The listing builds one solid part. Answer for the finished solid, in the listing's coordinates (mm). A direction names the side the tool comes from. Coordinates: 2 decimals unless noted, no trailing zeros. Loops run counter-clockwise (first coordinate to the right, second up) from the corner with the lowest first, then second, coordinate; pieces in that order, holes last. Notation, with made-up numbers: M 34,81 L 90,81 A10 cw 90,92 Z; hole C -1,-35 d11. An arc over 180 degrees is marked long. Answer as a JSON object with one key per item and string values. Group by question number.
1. A cutting plane is placed at B-B on x = 0. State how many separate pieces and enclosed holes the cut face has, and give its area (3 significant figures).
2. A cutting plane is placed at A-A on z = -19.05. Give the vertices of the cut face in (x, y) (3 decimals).
3. Straight lines are drawn through the part: L1, parallel to X at y = -11, z = 19; L2, parallel to X at y = 54, z = 12.5; L3, parallel to X at y = -44, z = 22. For each, find the intervals that lie inside material, in ascending order.
4. A cutting plane is placed at C-C on y = 31. Give the vertices of the cut face in (x, z).
5. Determine the mould class of faces 4 (the face through (0, -44, 19.3)), 5 (the face through (0, 1, 25.4)), 6 (the face through (0.044, -22.263, -18.706)) for opening direction Z: released by +Z, released by -Z, zero draft, split by the parting line, or undercut.
6. Given pin 1 (3 mm diameter, centred on x = 7.79, y = -31.24, fed in from +Z); pin 2 (2 mm diameter, centred on x = 14, z = 20.5, fed in from +Y); pin 3 (12 mm diameter, centred on x = -6, z = -10, fed in from +Y); pin 4 (8 mm diameter, centred on x = 13.5, z = 20.5, fed in from +Y), each flat-ended and moving along its own axis, determine where each tip first touches the part or whether it passes through.
7. For faces 1 (the face through (0, 56.059, 13)), 2 (the face through (12.7, 10, 12)), 3 (the face through (-8.11, -24.44, -12.52)), determine the directions among +Z, -Z, +X, -X, +Y, -Y from which every point of the face is accessible in a straight line to the end or side of a thin tool.
8. A cutting plane is placed at D-D on y = -39.5. Give the vertices of the cut face in (x, z), and give its area (3 significant figures).
from build123d import *

# Parameters (mm, degrees)
SKETCH1_R           = 4
SKETCH1_R_2         = 0.762
BOSS_EXTRUDE1_DEPTH = 25.4
SKETCH2_R           = 19.05
BOSS_EXTRUDE2_DEPTH = 25.4
SKETCH5_R           = 6.35
CUT_EXTRUDE2_DEPTH  = 25.4
SKETCH3_R           = 1.6
CUT_EXTRUDE1_DEPTH  = 25.4
SKETCH6_W           = 3.175
SKETCH6_H           = 1.5875
CUT_EXTRUDE3_DEPTH  = 25.4
SKETCH8_R           = 19.05
CUT_EXTRUDE4_DEPTH  = 19.3
BOSS_EXTRUDE3_DEPTH = 25.4
SKETCH10_W          = 6.35
SKETCH10_H          = 4.7625
BOSS_EXTRUDE4_DEPTH = 25.4
SKETCH11_R          = 1.5875
CUT_EXTRUDE5_DEPTH  = 23.225


with BuildPart() as part:
    # Sketch1 → Boss-Extrude1 (new body)
    with BuildSketch(Plane.XY):
        with BuildLine():
            Line((12.7, 50.8), (12.7, -50.8))
            ThreePointArc((12.7, -50.8), (0, -63.5), (-12.7, -50.8))
            Line((-12.7, -50.8), (-12.7, 50.8))
            ThreePointArc((-12.7, 50.8), (0, 63.5), (12.7, 50.8))
        make_face()
        with Locations((0, 50.8)):
            Circle(SKETCH1_R, mode=Mode.SUBTRACT)
        with Locations((-5.118745989, 55.918745989)):
            Circle(SKETCH1_R_2, mode=Mode.SUBTRACT)
        with Locations((5.118745989, 55.918745989)):
            Circle(SKETCH1_R_2, mode=Mode.SUBTRACT)
        with Locations((5.118745989, 45.681254011)):
            Circle(SKETCH1_R_2, mode=Mode.SUBTRACT)
        with Locations((-5.118745989, 45.681254011)):
            Circle(SKETCH1_R_2, mode=Mode.SUBTRACT)
    extrude(amount=BOSS_EXTRUDE1_DEPTH)

    # Sketch2 → Boss-Extrude2 (add)
    with BuildSketch(Plane(origin=(0, 0, 0), x_dir=(-1, 0, 0), z_dir=(0, 0, -1))):
        with Locations((0, -44.45)):
            Circle(SKETCH2_R)
    extrude(amount=-BOSS_EXTRUDE2_DEPTH)

    # Sketch5 → Cut-Extrude2 (cut)
    with BuildSketch(Plane.XY.offset(25.4)):
        with Locations((0, -51.562)):
            Circle(SKETCH5_R)
    extrude(amount=-CUT_EXTRUDE2_DEPTH, mode=Mode.SUBTRACT)

    # Sketch3 → Cut-Extrude1 (cut)
    with BuildSketch(Plane.XY.offset(25.4)):
        with Locations((-7.794229315, -31.235903463)):
            Circle(SKETCH3_R)
        with Locations((-15.2766, -44.45)):
            Circle(SKETCH3_R)
        with Locations((15.2766, -44.45)):
            Circle(SKETCH3_R)
        with Locations((-7.794229315, -58.017540858)):
            Circle(SKETCH3_R)
        with Locations((7.794229315, -31.235903463)):
            Circle(SKETCH3_R)
        with Locations((7.794229315, -58.017540858)):
            Circle(SKETCH3_R)
    extrude(amount=-CUT_EXTRUDE1_DEPTH, mode=Mode.SUBTRACT)

    # Sketch6 → Cut-Extrude3 (cut)
    with BuildSketch(Plane(origin=(0, 0, 0), x_dir=(-1, 0, 0), z_dir=(0, 0, -1))):
        with Locations((0, 55.265240671)):
            Rectangle(SKETCH6_W, SKETCH6_H)
    extrude(amount=-CUT_EXTRUDE3_DEPTH, mode=Mode.SUBTRACT)

    # Sketch8 → Cut-Extrude4 (cut)
    with BuildSketch(Plane(origin=(0, 0, 0), x_dir=(-1, 0, 0), z_dir=(0, 0, -1))):
        with Locations((0, -44.45)):
            Circle(SKETCH8_R)
    extrude(amount=-CUT_EXTRUDE4_DEPTH, mode=Mode.SUBTRACT)

    # Sketch9 → Boss-Extrude3 (add)
    with BuildSketch(Plane(origin=(0, 0, 0), x_dir=(-1, 0, 0), z_dir=(0, 0, -1))):
        with BuildLine():
            Line((-12.7, -30.250968343), (-12.7, -26.990386602))
            ThreePointArc((-12.7, -26.990386602), (0, -22.86), (12.7, -26.990386602))
            Line((12.7, -26.990386602), (12.7, -30.250968343))
            ThreePointArc((12.7, -30.250968343), (0, -25.4), (-12.7, -30.250968343))
        make_face()
    extrude(amount=BOSS_EXTRUDE3_DEPTH)

    # Sketch10 → Boss-Extrude4 (add)
    with BuildSketch(Plane(origin=(0, 0, 0), x_dir=(-1, 0, 0), z_dir=(0, 0, -1))):
        with Locations((0, -20.713481915)):
            Rectangle(SKETCH10_W, SKETCH10_H)
    extrude(amount=BOSS_EXTRUDE4_DEPTH)

    # Sketch11 → Cut-Extrude5 (cut, through all)
    with BuildSketch(Plane(origin=(3.175, 0, 0), x_dir=(0, 0, -1), z_dir=(1, 0, 0))):
        with Locations((6.35, -20.713481915)):
            Circle(SKETCH11_R)
        with Locations((19.05, -20.713481915)):
            Circle(SKETCH11_R)
    extrude(amount=-CUT_EXTRUDE5_DEPTH, mode=Mode.SUBTRACT)


solid = part.part
From the geometry:
{
 "1": {"separate pieces": "3", "enclosed holes": "2", "area": "2,340 mm²"},
 "2": {"outline": "M -12.7,-30.251 A19.05 cw 12.7,-30.251 L 12.7,-26.99 A21.59 ccw 3.175,-23.095 L 3.175,-22.301 L -3.175,-22.301 L -3.175,-23.095 A21.59 ccw -12.7,-26.99 Z; M -3.175,-19.126 L 3.175,-19.126 L 3.175,-18.332 L -3.175,-18.332 Z"},
 "3": {"L1": "x = -12.7 to 12.7", "L2": "x = -12.29 to -2.4, 2.4 to 12.29", "L3": "x = -19.04 to -16.81, -13.74 to 13.74, 16.81 to 19.04"},
 "4": {"outline": "M -12.7,0 L 12.7,0 L 12.7,25.4 L -12.7,25.4 Z"},
 "5": {"face 4": "released by -Z", "face 5": "released by +Z", "face 6": "undercut"},
 "6": {"pin 1": "passes through", "pin 2": "stops at y = -30.53", "pin 3": "stops at y = -18.33", "pin 4": "stops at y = 59.23"},
 "7": {"face 1": "+Z, -Z", "face 2": "+Z, -Z, +X, +Y", "face 3": "-Z, -X, +Y"},
 "8": {"outline": "M -18.4,19.3 L 18.4,19.3 L 18.4,25.4 L -18.4,25.4 Z", "area": "224 mm²"}
}
